Here's how the part is built. I have some questions about the finished solid (model axes, mm). A direction names the side the tool comes from. Coordinates: 2 decimals unless noted, no trailing zeros. Order: outer loops, then holes, each group sorted by start corner. A loop starts at its lowest first (then second) coordinate and runs counter-clockwise, first axis right, second up. Notation, with made-up numbers: (54, 16) -> (81, 16) arc R6 ccw to (81, 23) -> close; hole circle Ø8 at (-40, -1). An arc over 180 degrees is marked (long way). One line per item, written item: value. Start each with the question number.
```python
from build123d import *

# Parameters (mm, degrees)
SKETCH1_W           = 55.700676
SKETCH1_H           = 68.58
BOSS_EXTRUDE1_DEPTH = 3.175
SKETCH2_R           = 11.190499971
SKETCH2_R_2         = 1.5875
SKETCH2_R_3         = 1.397
SKETCH2_W           = 12.7
SKETCH2_H           = 7.9375
CUT_EXTRUDE1_DEPTH  = 89.407365824
SKETCH3_W           = 31.75
SKETCH3_H           = 1.905
CUT_EXTRUDE2_DEPTH  = 89.407365824
SKETCH4_R           = 1.778
CUT_EXTRUDE3_DEPTH  = 89.407365824
FILLET1_R           = 1.5875


with BuildPart() as part:
    # Sketch1 → Boss-Extrude1 (new body)
    with BuildSketch(Plane.XY):
        with Locations((27.850338, 34.29)):
            Rectangle(SKETCH1_W, SKETCH1_H)
    extrude(amount=BOSS_EXTRUDE1_DEPTH)

    # Sketch2 → Cut-Extrude1 (cut, through all)
    with BuildSketch(Plane.XY.offset(3.175)):
        with Locations((28.1492, 38.475)):
            Circle(SKETCH2_R)
        with Locations((12.6492, 53.975)):
            Circle(SKETCH2_R_2)
        with Locations((43.6492, 53.975)):
            Circle(SKETCH2_R_2)
        with Locations((43.6492, 22.975)):
            Circle(SKETCH2_R_2)
        with Locations((12.6492, 22.975)):
            Circle(SKETCH2_R_2)
        with Locations((17.4242, 17.005299976)):
            Circle(SKETCH2_R_3)
        with Locations((30.1242, 17.005299976)):
            Circle(SKETCH2_R_3)
        with Locations((23.7742, 3.96875)):
            Rectangle(SKETCH2_W, SKETCH2_H)
    extrude(amount=-CUT_EXTRUDE1_DEPTH, mode=Mode.SUBTRACT)

    # Sketch3 → Cut-Extrude2 (cut, through all)
    with BuildSketch(Plane.XY.offset(3.175)):
        with Locations((22.352, 0.9525)):
            Rectangle(SKETCH3_W, SKETCH3_H)
    extrude(amount=-CUT_EXTRUDE2_DEPTH, mode=Mode.SUBTRACT)

    # Sketch4 → Cut-Extrude3 (cut, through all)
    with BuildSketch(Plane.XY.offset(3.175)):
        with Locations((3, 55.88)):
            Circle(SKETCH4_R)
        with Locations((3, 25.4)):
            Circle(SKETCH4_R)
        with Locations((52.700676, 25.4)):
            Circle(SKETCH4_R)
        with Locations((52.700676, 55.88)):
            Circle(SKETCH4_R)
    extrude(amount=-CUT_EXTRUDE3_DEPTH, mode=Mode.SUBTRACT)

    # Fillet1
    fillet1_edges = [part.edges().sort_by_distance(p)[0] for p in [
        (17.4242, 7.9375, 1.5875),
        (30.1242, 7.9375, 1.5875),
        (6.477, 1.905, 1.5875),
        (38.227, 1.905, 1.5875),
    ]]
    fillet(fillet1_edges, radius=FILLET1_R)


solid = part.part
```
Q1. For faces 3 (the face through (13.503, 24.314, 1.61)), 4 (the face through (13, 1.905, 2)), which set-ups out of +Z, -Z, +X, -X, +Y, -Y let a thin tool reach every point of the face, with its end or its side?
Q2. Imagine slicing it at A-A (x = 3). Write out the boundary of the cut face in (y, z) (3 decimals), plus the area to 3 significant figures.
Q3. Imagine slicing it at C-C (z = 1.65). Count the separate pieces of the cut face and the enclosed holes in it, plus the area to 3 significant figures.
Q4. Imagine slicing it at B-B (y = 25.4). Write out the boundary of the cut face in (x, z) (3 decimals), plus the area to 3 significant figures.
Q5. Imagine slicing it at D-D (y = 35). Write out the boundary of the cut face in (x, z) (3 decimals).
Q6. I need wall thicknesses on line 1 (X direction, y = 22, z = 0.9); line 2 (Y direction, x = 18.5, z = 0.2); line 3 (Y direction, x = 13, z = 0.85) (3 decimals). Which ranges of each line are inside material? Lowest first, please.
Q7. If we mould it in two halves opening along X, with no side actions, what happens to faces 1 (the face through (27, 27, 3.175)), 2 (the face through (17.877, 7.46, 1.565))? For each: +X half, -X half, draft (parallel to the pull), parting line (faces both ways), or undercut.
Q8. For P1, Ø1.5, axis at x = 8, z = 0.5, coming from the -Y side; P2, Ø1.6, axis at x = 14.5, z = 2, coming from the -Y side (3 decimals); P3, Ø5.5, axis at x = 52.7, y = 25.4, coming from the +Z side (3 decimals), each with a flat end and sliding along its axis, tell me the tip position at first contact or that it passes through.
Completed:
1. face 3: +Z, -Z
1. face 4: +Z, -Z, -Y
2. outline: (0, 0) -> (23.622, 0) -> (23.622, 3.175) -> (0, 3.175) -> close; (27.178, 0) -> (54.102, 0) -> (54.102, 3.175) -> (27.178, 3.175) -> close; (57.658, 0) -> (68.58, 0) -> (68.58, 3.175) -> (57.658, 3.175) -> close
2. area: 195 mm2
3. separate pieces: 1
3. enclosed holes: 11
3. area: 3,210 mm2
4. outline: (0, 0) -> (1.222, 0) -> (1.222, 3.175) -> (0, 3.175) -> close; (4.778, 0) -> (50.923, 0) -> (50.923, 3.175) -> (4.778, 3.175) -> close; (54.479, 0) -> (55.701, 0) -> (55.701, 3.175) -> (54.479, 3.175) -> close
4. area: 154 mm2
5. outline: (0, 0) -> (17.512, 0) -> (17.512, 3.175) -> (0, 3.175) -> close; (38.786, 0) -> (55.701, 0) -> (55.701, 3.175) -> (38.786, 3.175) -> close
6. line 1: x = 0 to 11.4, 13.9 to 42.4, 44.9 to 55.7
6. line 2: y = 7.85 to 16.11, 17.9 to 32.81, 44.14 to 68.58
6. line 3: y = 1.905 to 21.427, 24.523 to 52.427, 55.523 to 68.58
7. face 1: draft
7. face 2: undercut
8. P1: stops at y = 1.68
8. P2: stops at y = 1.905
8. P3: stops at z = 3.175
